Read the model definition and answer for the solid it produces. Units are mm, in the model's axes. Face numbers are marked on the shaded views. Coordinates: 2 decimals unless noted, no trailing zeros. Write each loop counter-clockwise with the first axis right and the second up, starting at its lowest first coordinate (ties: lowest second). Pieces come first, ordered by that corner, then holes. Notation, with made-up numbers: (85, 56.5) -> (140, 56.5) arc R22 ccw to (140, 89.5) -> close; hole circle Ø5 at (80, 36.25). An arc over 180 degrees is marked (long way). Write item = value, one per line. Start each with the question number.
1) Section A-A (x = 0) is taken. Determine the outline of the cut face in (y, z), plus the area to 3 significant figures.
2) Find the intervals of material crossed by line 1 along Y through (x, z) = (0, 14.5); line 2 along Y through (x, z) = (0, 3.75); line 3 along Z through (x, y) = (-2.25, 2), in increasing order. Write a range as from..to.
3) Flat-ended cylindrical pins translate along their axes: pin 1 Ø1.5 at (x, y) = (0.5, -1) entering from -Z; pin 2 Ø2 at (y, z) = (-1, 7.5) entering from -X; pin 3 Ø2 at (x, y) = (0, 0) entering from -Z. Find the tip coordinate at first contact, or state that the pin passes through.
4) Section C-C (z = 4.25) is taken. Determine the outline of the cut face in (x, y).
5) Section D-D (y = 3.25) is taken. Determine the outline of the cut face in (x, z).
6) For a pull along X with two mould halves and no side action, classify the marked faces 1, 2, 3 and 4 as released by +X, released by -X, zero draft, split by the parting line, or undercut.
from build123d import *


with BuildPart() as f1:
    # F0 (on Front) → F1 (revolve)
    with BuildSketch(Plane.XZ):
        Polygon((-3.8, 0), (-2.8, 0), (-2.8, 6.45), (-2.8, 8), (-1.25, 8), (-1.25, 23), (-2.25, 23), (-2.25, 9), (-3.8, 9), align=None)
        Polygon((-2.8, 8), (-2.8, 6.45), (-1.25, 8), align=None)
    revolve(axis=Axis((0, 0, 11.5), (0, 0, -1)))


solid = f1.part
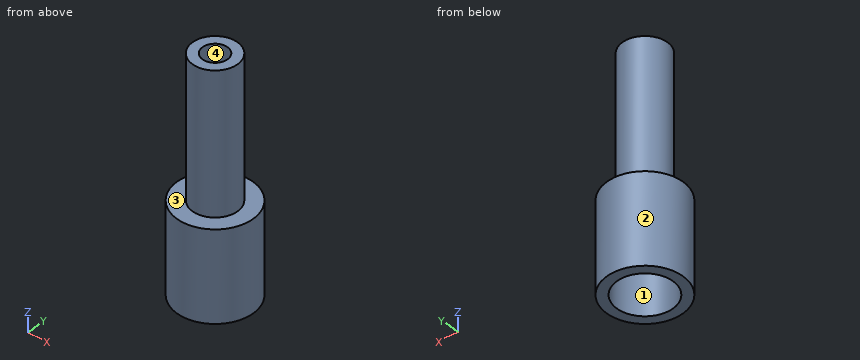
Answer key:
q1.outline = (-3.8, 0) -> (-2.8, 0) -> (-2.8, 6.45) -> (-1.25, 8) -> (-1.25, 23) -> (-2.25, 23) -> (-2.25, 9) -> (-3.8, 9) -> close; (1.25, 8) -> (2.8, 6.45) -> (2.8, 0) -> (3.8, 0) -> (3.8, 9) -> (2.25, 9) -> (2.25, 23) -> (1.25, 23) -> close
q1.area = 51.5 mm^2
q2.line_1 = -2.25..-1.25, 1.25..2.25
q2.line_2 = -3.8..-2.8, 2.8..3.8
q2.line_3 = 0..9
q3.pin_1 = 7.38
q3.pin_2 = -3.8
q3.pin_3 = through
q4.outline = circle Ø7.6 at (0, 0); hole circle Ø5.6 at (0, 0)
q5.outline = (-1.97, 0) -> (1.97, 0) -> (1.97, 9) -> (-1.97, 9) -> close
q6.face_1 = undercut
q6.face_2 = split by the parting line
q6.face_3 = zero draft
q6.face_4 = undercut
